CAD build for the part. Positions are in the model's coordinates, mm. A direction names the side the tool comes from. Round coordinates to 2 decimals unless told otherwise and drop trailing zeros. Write each loop counter-clockwise with the first axis right and the second up, starting at its lowest first coordinate (ties: lowest second). Pieces come first, ordered by that corner, then holes. Notation, with made-up numbers: (76.25, -29.75) - (133.25, -29.75) arc R36 ccw to (133.25, 7.25) - close; hole circle Ø2 at (-40, 42.25). An arc over 180 degrees is marked (long way). Put each result on its own line as item: value. Start each with the question number.
Item 1: Cut at C-C (y = 86.5). Give the cut face in (x, z), and give its area (3 significant figures).
Item 2: Mould opens along Y. For faces 1 (the cylindrical face through (13.72, 23.11, 5.07)), 2 (the flat face through (24, 74, 5)), 3 (the cylindrical face through (-33.002, 68.755, 4.93)), 4 (the cylindrical face through (33.002, 68.755, 4.93)) say: released by +Y, released by -Y, zero draft, split by the parting line, or undercut.
Item 3: Cut at A-A (y = 70). Give the cut face in (x, z), and give its area (3 significant figures).
Item 4: Pin check, flat tip, straight feed: pin 1 Ø5 at (x, z) = (8.5, 4.5) entering from +Y. Stop position of the tip, or through.
Item 5: 3-axis set-ups, long thin cutter, end or side, ignore diameter. For faces 5 (the cylindrical face through (-31.5, 101.117, 4.93)), 6 (the flat face through (-24, 74, 5)), 7 (the cylindrical face through (16.778, 16.938, 5.07)): which of +Z, -Z, +X, -X, +Y, -Y reach the whole face in a straight line?
Item 6: Cut at D-D (x = -30). Give the cut face in (y, z).
Item 7: Cut at B-B (z = 7.75). Give the cut face in (x, y), and give its area (3 significant figures).
Item 8: Drill centre lines: line 1 (Y direction, x = 22, z = 6.5); line 2 (X direction, y = 21, z = 9); line 3 (X direction, y = 99, z = 7). Where is each one in solid material? Low to high. Write a range as from..to.
```python
from build123d import *

# Parameters (mm, degrees)
ESQUISSE1_R        = 3.25
ESQUISSE1_R_2      = 3.5
BOSS_EXTRU_1_DEPTH = 10
CONG_1_R           = 4
CONG_2_R           = 8
CONG_3_R           = 7


with BuildPart() as part:
    # Esquisse1 → Boss.-Extru.1 (new body)
    with BuildSketch(Plane.XY):
        Polygon((24, 110), (24, 36), (0, 36), (0, 24), (14.5, 24), (16.055042473, 16), (36, 16), (36, 110), align=None)
        with Locations((30, 104)):
            Circle(ESQUISSE1_R, mode=Mode.SUBTRACT)
        with Locations((22, 23)):
            Circle(ESQUISSE1_R_2, mode=Mode.SUBTRACT)
        with Locations((30, 70)):
            Circle(ESQUISSE1_R, mode=Mode.SUBTRACT)
    boss_extru_1 = extrude(amount=BOSS_EXTRU_1_DEPTH)

    # Symétrie2: Boss.-Extru.1 across plane
    add(boss_extru_1.mirror(Plane(origin=(0, 36, 10), x_dir=(0, 0, 1), z_dir=(1, 0, 0))))

    # Congé1
    cong_1_edges = [part.edges().sort_by_distance(p)[0] for p in [
        (16.055042473, 16, 5),
        (14.5, 24, 5),
        (-14.5, 24, 5),
        (-16.055042473, 16, 5),
    ]]
    fillet(cong_1_edges, radius=CONG_1_R)

    # Congé2
    cong_2_edges = [part.edges().sort_by_distance(p)[0] for p in [
        (36, 16, 5),
        (-36, 16, 5),
    ]]
    fillet(cong_2_edges, radius=CONG_2_R)

    # Congé3
    cong_3_edges = [part.edges().sort_by_distance(p)[0] for p in [
        (36, 110, 5),
        (-36, 110, 5),
    ]]
    fillet(cong_3_edges, radius=CONG_3_R)


solid = part.part
```
Output values:
1. outline: (-36, 0) - (-24, 0) - (-24, 10) - (-36, 10) - close; (24, 0) - (36, 0) - (36, 10) - (24, 10) - close
1. area: 240 mm2
2. face 1: released by -Y
2. face 2: zero draft
2. face 3: undercut
2. face 4: undercut
3. outline: (-36, 0) - (-33.25, 0) - (-33.25, 10) - (-36, 10) - close; (-26.75, 0) - (-24, 0) - (-24, 10) - (-26.75, 10) - close; (24, 0) - (26.75, 0) - (26.75, 10) - (24, 10) - close; (33.25, 0) - (36, 0) - (36, 10) - (33.25, 10) - close
3. area: 110 mm2
4. pin 1: y = 36
5. face 5: +Z, -Z
5. face 6: +Z, -Z, +Y
5. face 7: +Z, -Z, -Y
6. outline: (16.25, 0) - (66.75, 0) - (66.75, 10) - (16.25, 10) - close; (73.25, 0) - (100.75, 0) - (100.75, 10) - (73.25, 10) - close; (107.25, 0) - (109.93, 0) - (109.93, 10) - (107.25, 10) - close
7. outline: (-36, 24) arc R8 ccw to (-28, 16) - (-19.35, 16) arc R4 ccw to (-15.43, 19.24) - (-15.13, 20.76) arc R4 cw to (-11.2, 24) - (11.2, 24) arc R4 cw to (15.13, 20.76) - (15.43, 19.24) arc R4 ccw to (19.35, 16) - (28, 16) arc R8 ccw to (36, 24) - (36, 103) arc R7 ccw to (29, 110) - (24, 110) - (24, 36) - (-24, 36) - (-24, 110) - (-29, 110) arc R7 ccw to (-36, 103) - close; hole circle Ø6.5 at (-30, 70); hole circle Ø6.5 at (-30, 104); hole circle Ø7 at (-22, 23); hole circle Ø7 at (22, 23); hole circle Ø6.5 at (30, 70); hole circle Ø6.5 at (30, 104)
7. area: 2,710 mm2
8. line 1: 16..19.5, 26.5..36
8. line 2: -35.42..-24.87, -19.13..-15.08, 15.08..19.13, 24.87..35.42
8. line 3: -36..-24, 24..36
